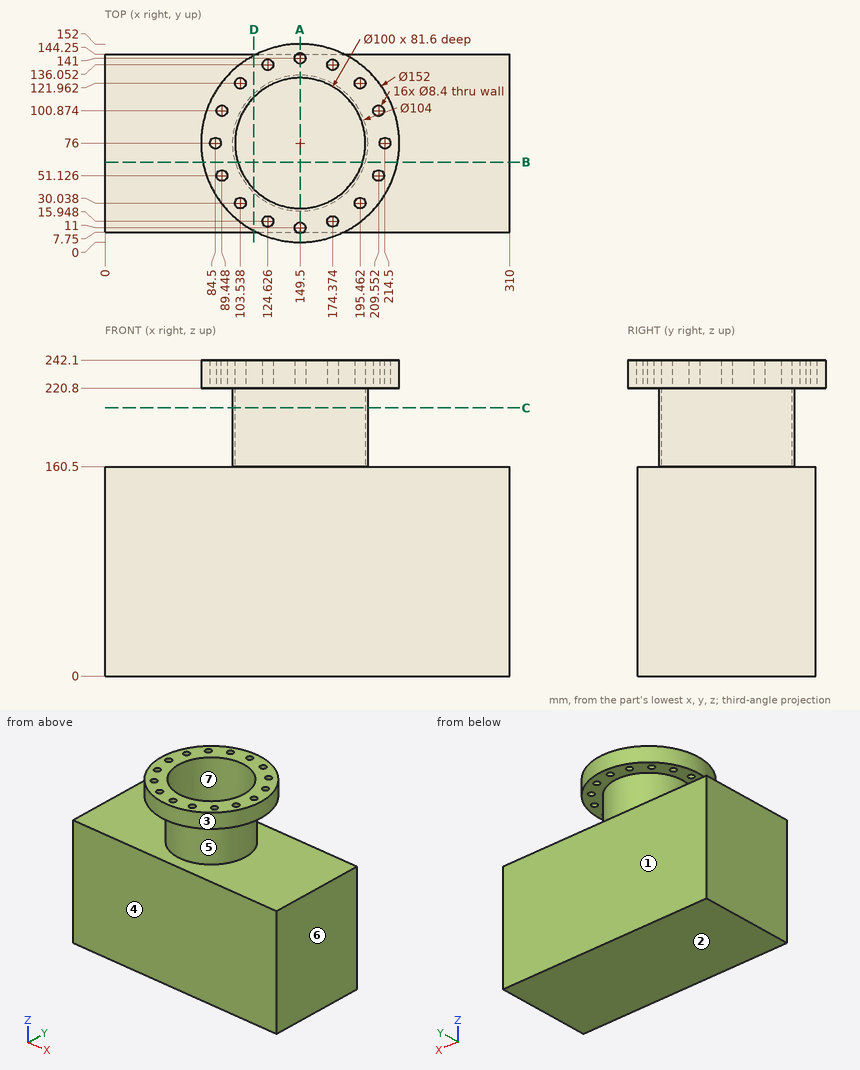
Input: dimensioned drawing with shaded views. Units: mm. Origin: part minimum x, y, z. A direction names the side the tool comes from. Coordinates: 2 decimals unless noted, no trailing zeros. Write each loop counter-clockwise with the first axis right and the second up, starting at its lowest first coordinate (ties: lowest second). Pieces come first, ordered by that corner, then holes. Notation, with made-up numbers: M -10.5,30 L 44.5,30 A12 cw 44.5,36 Z; hole C 62.25,38.25 d1. An arc over 180 degrees is marked long. Use a Markdown table: item, result.
1) Mould query, pull axis Y, two halves, no side actions, for the marked faces 4, 5, 6 and 7. Classes: pulls with the +Y half, pulls with the -Y half, needs draft (parallel to the pull), parting line crosses it, or undercut.
Conclusion:
| item | result |
|---|---|
| face 4 | pulls with the -Y half |
| face 5 | parting line crosses it |
| face 6 | needs draft |
| face 7 | undercut |
2) Section B-B, the plane y = 61.5. Output: boundary loops of the cut face in (x, z).
Conclusion:
| item | result |
|---|---|
| outline | M 0,0 L 310,0 L 310,160.5 L 199.44,160.5 L 199.44,220.8 L 224.1,220.8 L 224.1,242.1 L 197.35,242.1 L 197.35,160.5 L 101.65,160.5 L 101.65,242.1 L 74.9,242.1 L 74.9,220.8 L 99.56,220.8 L 99.56,160.5 L 0,160.5 Z |
3) Ray query, L1, parallel to Z at x = 196, y = 116.5; L2, parallel to X at y = 77, z = 180.5; L3, parallel to Z at x = 109.5, y = 9. Return the intervals inside material, ascending.
Conclusion:
| item | result |
|---|---|
| L1 | z = 0 to 160.5, 220.8 to 242.1 |
| L2 | x = 97.51 to 99.51, 199.49 to 201.49 |
| L3 | z = 0 to 160.5 |
4) Section D-D, the plane x = 114. Output: boundary loops of the cut face in (y, z).
Conclusion:
| item | result |
|---|---|
| outline | M 7.75,0 L 144.25,0 L 144.25,160.5 L 114,160.5 L 114,220.8 L 143.2,220.8 L 143.2,242.1 L 111.21,242.1 L 111.21,160.5 L 40.79,160.5 L 40.79,242.1 L 8.8,242.1 L 8.8,220.8 L 38,220.8 L 38,160.5 L 7.75,160.5 Z |
5) First-contact query: pin 1 Ø8 at (x, z) = (50.5, 149.5) entering from -Y; pin 2 Ø10 at (x, y) = (177, 100) entering from +Z; pin 3 Ø8 at (x, z) = (102, 153.5) entering from +Y. Flat tips, straight axial feed; report the tip coordinate or a pass-through.
Conclusion:
| item | result |
|---|---|
| pin 1 | stops at y = 7.75 |
| pin 2 | stops at z = 160.5 |
| pin 3 | stops at y = 144.25 |
6) Section A-A, the plane x = 149.5. Output: boundary loops of the cut face in (y, z), then the cut area to 3 significant figures.
Conclusion:
| item | result |
|---|---|
| outline | M 0,220.8 L 6.8,220.8 L 6.8,242.1 L 0,242.1 Z; M 7.75,0 L 144.25,0 L 144.25,160.5 L 128,160.5 L 128,220.8 L 136.8,220.8 L 136.8,242.1 L 126,242.1 L 126,160.5 L 26,160.5 L 26,242.1 L 15.2,242.1 L 15.2,220.8 L 24,220.8 L 24,160.5 L 7.75,160.5 Z; M 145.2,220.8 L 152,220.8 L 152,242.1 L 145.2,242.1 Z |
| area | 22,900 mm^2 |
7) Section C-C, the plane z = 205.5. Output: boundary loops of the cut face in (x, y).
Conclusion:
| item | result |
|---|---|
| outline | C 149.5,76 d104; hole C 149.5,76 d100 |
8) Reachability of the marked faces 1, 2 and 3 from +Z, -Z, +X, -X, +Y, -Y: full face, straight path, thin tool, end or side. Return the list, or none.
Conclusion:
| item | result |
|---|---|
| face 1 | -Z, +X, -X, +Y |
| face 2 | -Z, +X, -X, +Y, -Y |
| face 3 | +Z |
